Build history of the part. All positions in model axes, mm. A direction names the side the tool comes from. Round coordinates to 2 decimals unless told otherwise and drop trailing zeros. Write each loop counter-clockwise with the first axis right and the second up, starting at its lowest first coordinate (ties: lowest second). Pieces come first, ordered by that corner, then holes. Notation, with made-up numbers: (21.5, 17.25) -> (44.5, 17.25) arc R7 cw to (44.5, 21.25) -> close; hole circle Ø8 at (53.5, 16.5). An arc over 180 degrees is marked (long way). Answer in a Markdown table with one row per item.
```python
from build123d import *

# Parameters (mm, degrees)
SKETCH1_R      = 7.5
EXTRUDE1_DEPTH = 36.5
SKETCH2_W      = 32
SKETCH2_H      = 21
EXTRUDE2_DEPTH = 5.5
SKETCH3_R      = 4
EXTRUDE3_DEPTH = 42
SKETCH4_R      = 21
SKETCH4_R_2    = 16
EXTRUDE4_DEPTH = 10
SKETCH5_R      = 6.8
SKETCH5_R_2    = 4.6
EXTRUDE5_DEPTH = 0.3
EXTRUDE6_START = -0.3
SKETCH6_R      = 6.8
SKETCH6_R_2    = 4.6
EXTRUDE6_DEPTH = 0.3
SKETCH7_W      = 0.2
SKETCH7_H      = 1
SKETCH8_R      = 1.5
EXTRUDE7_DEPTH = 8
SKETCH8_3_R    = 2.75
EXTRUDE8_DEPTH = 3.5
CHAMFER1_SIZE  = 0.2


with BuildPart() as part:
    # Sketch1 → Extrude1 (new body)
    with BuildSketch(Plane(origin=(0, 0, 0), x_dir=(1, 0, 0), z_dir=(0, 1, 0))):
        with Locations(Location((0, 0, 0), (0, 0, 270))):
            Circle(SKETCH1_R)
    extrude(amount=EXTRUDE1_DEPTH)

    # Sketch2 → Extrude2 (add)
    with BuildSketch(Plane(origin=(0, 36.5, 0), x_dir=(1, 0, 0), z_dir=(0, 1, 0))):
        Rectangle(SKETCH2_W, SKETCH2_H)
    extrude(amount=EXTRUDE2_DEPTH)

    # Sketch3 → Extrude3 (cut)
    with BuildSketch(Plane.XZ):
        with Locations(Location((0, 0, 0), (0, 0, 270))):
            Circle(SKETCH3_R)
    extrude(amount=-EXTRUDE3_DEPTH, mode=Mode.SUBTRACT)

    # Sketch4 → Extrude4 (cut)
    with BuildSketch(Plane(origin=(0, 42, 0), x_dir=(1, 0, 0), z_dir=(0, 1, 0))):
        Circle(SKETCH4_R)
        Circle(SKETCH4_R_2, mode=Mode.SUBTRACT)
    extrude(amount=-EXTRUDE4_DEPTH, mode=Mode.SUBTRACT)

    # Sketch5 → Extrude5 (cut)
    with BuildSketch(Plane.XZ):
        with Locations(Location((0, 0, 0), (0, 0, 270))):
            Circle(SKETCH5_R)
        with Locations(Location((0, 0, 0), (0, 0, 270))):
            Circle(SKETCH5_R_2, mode=Mode.SUBTRACT)
    extrude(amount=-EXTRUDE5_DEPTH, mode=Mode.SUBTRACT)

    # Sketch6 → Extrude6 (cut)
    with BuildSketch(Plane(origin=(0, 42, 0), x_dir=(1, 0, 0), z_dir=(0, 1, 0)).offset(EXTRUDE6_START)):
        with Locations(Location((0, 0, 0), (0, 0, 90))):
            Circle(SKETCH6_R)
        with Locations(Location((0, 0, 0), (0, 0, 90))):
            Circle(SKETCH6_R_2, mode=Mode.SUBTRACT)
    extrude(amount=EXTRUDE6_DEPTH, mode=Mode.SUBTRACT)

    # Sketch7 → Cut-Revolve1 (revolve, cut)
    with BuildSketch(Plane(origin=(0, 0, 0), x_dir=(0, 0, -1), z_dir=(1, 0, 0))):
        with Locations((7.4, 3.5)):
            Rectangle(SKETCH7_W, SKETCH7_H)
    revolve(axis=Axis((0, 0, 0), (0, 1, 0)), mode=Mode.SUBTRACT)

    # Sketch8 → Extrude7 (cut)
    with BuildSketch(Plane(origin=(0, 42, 0), x_dir=(1, 0, 0), z_dir=(0, 1, 0))):
        with Locations(Location((-12.25, 0, 0), (0, 0, 270))):
            Circle(SKETCH8_R)
        with Locations(Location((12.25, 0, 0), (0, 0, 270))):
            Circle(SKETCH8_R)
    extrude(amount=-EXTRUDE7_DEPTH, mode=Mode.SUBTRACT)

    # Sketch8_3 → Extrude8 (cut)
    with BuildSketch(Plane(origin=(0, 42, 0), x_dir=(1, 0, 0), z_dir=(0, 1, 0))):
        with Locations(Location((-12.25, 0, 0), (0, 0, 270))):
            Circle(SKETCH8_3_R)
        with Locations(Location((12.25, 0, 0), (0, 0, 270))):
            Circle(SKETCH8_3_R)
    extrude(amount=-EXTRUDE8_DEPTH, mode=Mode.SUBTRACT)

    # Chamfer1
    chamfer1_edges = [part.edges().sort_by_distance(p)[0] for p in [
        (0, 42, 4),
        (0, 0, 4),
        (0, 0, -7.5),
        (0, 0, 6.8),
        (0, 0, 4.6),
        (0, 42, 6.8),
        (0, 42, 4.6),
    ]]
    chamfer(chamfer1_edges, length=CHAMFER1_SIZE)


solid = part.part
```
Q1. Saw through at C-C on z = 0. State how many separate pieces and enclosed holes the cut face has, plus the area to 3 significant figures.
A:
| item | result |
|---|---|
| separate pieces | 4 |
| enclosed holes | 0 |
| area | 334 mm² |
Q2. Saw through at B-B on y = 35. Write the cut outline in (x, z), plus the area to 3 significant figures.
A:
| item | result |
|---|---|
| outline | circle Ø15 at (0, 0); hole circle Ø8 at (0, 0) |
| area | 126 mm² |
Q3. Which spindle directions (+Z, -Z, +X, -X, +Y, -Y) get a long thin tool onto all of the face, cutting with end or side? Do faces 5 (the cylindrical face through (-16, 39, 0)), 6 (the flat face through (-13.4, 38.5, 1.2)). Say none if no direction does.
A:
| item | result |
|---|---|
| face 5 | -X, +Y, -Y |
| face 6 | +Y |
Q4. Drop flat-ended pins along their axis: P1, Ø8, axis at y = 8.5, z = -1.5, coming from the +X side; P2, Ø4, axis at x = 12.25, z = 0, coming from the +Y side; P3, Ø10, axis at x = -5, y = 30, coming from the +Z side. Give the stop position or say it passes through.
A:
| item | result |
|---|---|
| P1 | x = 7.5 |
| P2 | y = 38.5 |
| P3 | z = 7.5 |
Q5. Two-plate mould, pull along X, no slides. Class faces 1 (the cylindrical face through (16, 39, 0)), 2 (the flat face through (-7.34, 36.5, 2.19)), 3 (the flat face through (11.1, 38.5, 1.2)), 4 (the cylindrical face through (12.7, 37.51, 1.43)): released by +X, released by -X, zero draft, split by the parting line, or undercut.
A:
| item | result |
|---|---|
| face 1 | released by +X |
| face 2 | zero draft |
| face 3 | undercut |
| face 4 | undercut |
Q6. Saw through at A-A on x = -11.5. Write the cut outline in (y, z), plus the area to 3 significant figures.
A:
| item | result |
|---|---|
| outline | (36.5, -10.5) -> (42, -10.5) -> (42, -2.65) -> (38.5, -2.65) -> (38.5, -1.3) -> (36.5, -1.3) -> close; (36.5, 1.3) -> (38.5, 1.3) -> (38.5, 2.65) -> (42, 2.65) -> (42, 10.5) -> (36.5, 10.5) -> close |
| area | 91.8 mm² |
Q7. Wall check: line 1 (X direction, y = 37.55, z = 0); line 2 (Z direction, x = 12, y = 40); line 3 (X direction, y = 39.35, z = 0). Give the ranges that are in metal, low to high. Write a range as [from, to].
A:
| item | result |
|---|---|
| line 1 | [-16, -13.75], [-10.75, -4], [4, 10.75], [13.75, 16] |
| line 2 | [-10.5, -2.74], [2.74, 10.5] |
| line 3 | [-16, -15], [-9.5, -4], [4, 9.5], [15, 16] |
